Design review of the part built by this model. Coordinates are the model's own, in mm. Face numbers are marked on the shaded views. Coordinates: 2 decimals unless noted, no trailing zeros. Write each loop counter-clockwise with the first axis right and the second up, starting at its lowest first coordinate (ties: lowest second). Pieces come first, ordered by that corner, then holes. Notation, with made-up numbers: (-29, 54.5) -> (1, 54.5) arc R20 cw to (1, 90.5) -> close; hole circle Ø5 at (65, 21.25). An arc over 180 degrees is marked (long way). One line per question, with ' | ' between items. Start each with the question number.
Q1. For P1, Ø1.7, axis at x = 51, z = -55.5, coming from the +Y side; P2, Ø3, axis at x = 9.56, z = -17.28, coming from the +Y side; P3, Ø5.5, axis at x = 51.46, z = -30.78, coming from the -Y side; P4, Ø1.2, axis at x = 22.5, y = 2.5, coming from the -Z side, all flat-tipped, find the tip position at first contact; note any pin that passes through.
Q2. Add section A-A on z = -41.5. State the section outline as (x, y) points.
Q3. Draft analysis for pull direction Y (two halves, no side actions). For the marked faces 1 and 2, state which applies: pulls with the +Y half, pulls with the -Y half, needs draft (parallel to the pull), parting line crosses it, or undercut.
Q4. Wall thickness on probe 1 along X at (y, z) = (1.8, -15); probe 2 along X at (y, z) = (0.4, -55.5); probe 3 along X at (y, z) = (1.5, -41.5): over which ranges is each line inside the solid? List them lowest first.
Q5. Add section B-B on y = 2.65. State the section outline as (x, z) points.
Q6. Add section D-D on z = -18. State the section outline as (x, y) points, and give its area (3 significant figures).
Q7. Add section C-C on x = 21. State the section outline as (y, z) points.
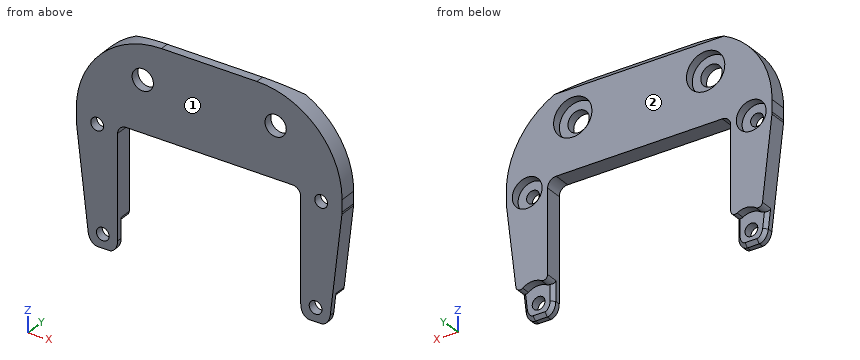
from build123d import *

# Parameters (mm, degrees)
SZKIC1_R                    = 1.5
SZKIC1_R_2                  = 2.5
DODANIE_WYCI_GNI_CIE1_DEPTH = 4
ZAOKR_GLENIE1_R             = 20
SZKIC2_R                    = 3.5
SZKIC2_R_2                  = 4
SZKIC2_R_3                  = 4.5
WYTNIJ_WYCI_GNI_CIE1_DEPTH  = 2
ZAOKR_GLENIE2_R             = 1
SFAZOWANIE2_SIZE            = 0.8


with BuildPart() as part:
    # Szkic1 → Dodanie-wyciągnięcie1 (new body)
    with BuildSketch(Plane(origin=(0, 0, 0), x_dir=(1, 0, 0), z_dir=(0, 1, 0))):
        with BuildLine():
            Line((1.659006671, 58.277593275), (-1.119868317, 58.277593275))
            add(Edge.make_bspline(
                [(-1.119868317, 58.277593275), (-2.968900305, 58.277593275), (-3.270926516, 55.680167866)],
                knots=[3.223355162, 3.223355162, 3.223355162, 4.71238898, 4.71238898, 4.71238898], degree=2, weights=[1, 0.735415338, 1]))
            Line((-3.270926516, 55.680167866), (-6.019830139, 32.039596707))
            ThreePointArc((-6.019830139, 32.039596707), (-6.039902389, 31.808982465), (-6.046600617, 31.577593275))
            Line((-6.046600617, 31.577593275), (-6.046600617, 8.777593275))
            Line((-6.046600617, 8.777593275), (56.36461396, 8.777593275))
            Line((56.36461396, 8.777593275), (56.36461396, 31.577593275))
            ThreePointArc((56.36461396, 31.577593275), (56.357915732, 31.808982465), (56.337843482, 32.039596707))
            Line((56.337843482, 32.039596707), (53.588939858, 55.680167866))
            add(Edge.make_bspline(
                [(53.588939858, 55.680167866), (53.286913648, 58.277593275), (51.43788166, 58.277593275)],
                knots=[1.570796327, 1.570796327, 1.570796327, 3.059830145, 3.059830145, 3.059830145], degree=2, weights=[1, 0.735415338, 1]))
            Line((51.43788166, 58.277593275), (48.659006671, 58.277593275))
            add(Edge.make_bspline(
                [(48.659006671, 58.277593275), (46.659006671, 58.277593275), (46.659006671, 55.44916615)],
                knots=[3.141592654, 3.141592654, 3.141592654, 4.71238898, 4.71238898, 4.71238898], degree=2, weights=[1, 0.707106781, 1]))
            Line((46.659006671, 55.44916615), (46.659006671, 31.277593275))
            ThreePointArc((46.659006671, 31.277593275), (46.073220234, 29.863379712), (44.659006671, 29.277593275))
            Line((44.659006671, 29.277593275), (5.659006671, 29.277593275))
            ThreePointArc((5.659006671, 29.277593275), (4.244793109, 29.863379712), (3.659006671, 31.277593275))
            Line((3.659006671, 31.277593275), (3.659006671, 55.44916615))
            add(Edge.make_bspline(
                [(3.659006671, 55.44916615), (3.659006671, 58.277593275), (1.659006671, 58.277593275)],
                knots=[1.570796327, 1.570796327, 1.570796327, 3.141592654, 3.141592654, 3.141592654], degree=2, weights=[1, 0.707106781, 1]))
        make_face()
        with Locations(Location((50.145621432, 55.076817676, 0), (0, 0, 270))):
            Circle(SZKIC1_R, mode=Mode.SUBTRACT)
        with Locations(Location((0.172391911, 55.076817676, 0), (0, 0, 270))):
            Circle(SZKIC1_R, mode=Mode.SUBTRACT)
        with Locations(Location((-1.144922446, 30.775394297, 0), (0, 0, 270))):
            Circle(SZKIC1_R, mode=Mode.SUBTRACT)
        with Locations(Location((51.462935789, 30.775394297, 0), (0, 0, 270))):
            Circle(SZKIC1_R, mode=Mode.SUBTRACT)
        with Locations(Location((40.761810316, 17.277593275, 0), (0, 0, 270))):
            Circle(SZKIC1_R_2, mode=Mode.SUBTRACT)
        with Locations(Location((9.556203027, 17.277593275, 0), (0, 0, 90))):
            Circle(SZKIC1_R_2, mode=Mode.SUBTRACT)
    extrude(amount=DODANIE_WYCI_GNI_CIE1_DEPTH)

    # Zaokrąglenie1
    zaokr_glenie1_edges = [part.edges().sort_by_distance(p)[0] for p in [
        (56.36461396, 2, -8.777593275),
        (-6.046600617, 2, -8.777593275),
    ]]
    fillet(zaokr_glenie1_edges, radius=ZAOKR_GLENIE1_R)

    # Szkic2 → Wytnij-wyciągnięcie1 (cut)
    with BuildSketch(Plane(origin=(0, 4, 0), x_dir=(1, 0, 0), z_dir=(0, 1, 0))):
        with Locations(Location((51.462935789, 30.775394297, 0), (0, 0, 270))):
            Circle(SZKIC2_R)
        with Locations((50.145621432, 55.076817676)):
            Circle(SZKIC2_R_2)
        with Locations((0.172391911, 55.076817676)):
            Circle(SZKIC2_R_2)
        with Locations(Location((-1.144922446, 30.775394297, 0), (0, 0, 270))):
            Circle(SZKIC2_R)
        with Locations(Location((9.556203027, 17.277593275, 0), (0, 0, 270))):
            Circle(SZKIC2_R_3)
        with Locations(Location((40.761810316, 17.277593275, 0), (0, 0, 270))):
            Circle(SZKIC2_R_3)
    extrude(amount=-WYTNIJ_WYCI_GNI_CIE1_DEPTH, mode=Mode.SUBTRACT)

    # Zaokrąglenie2
    zaokr_glenie2_edges = [part.edges().sort_by_distance(p)[0] for p in [
        (53.837974946, 3, -53.538466114),
        (-3.519961603, 3, -53.538466114),
        (3.659006671, 3, -53.116328576),
        (46.659006671, 3, -53.116328576),
    ]]
    fillet(zaokr_glenie2_edges, radius=ZAOKR_GLENIE2_R)

    # Sfazowanie1
    # the kernel refuses this chamfer: 2 mm, written as the material it takes off along each edge
    with BuildSketch(Plane(origin=(1.60932104, 4, -8.777593275), x_dir=(0, 0.027495876610586487, -0.9996219169112968), z_dir=(1, 0, 0))) as sfazowanie1_piece_1:
        with BuildLine():
            Line((2.05734639, 0), (-0.11309431, -2.054235587))
            Line((-0.11309431, -2.054235587), (-0.153079186, -2.053135752))
            ThreePointArc((-0.153079186, -2.053135752), (-0.068258454, -1.026795659), (-0.039984877, 0.001099835))
            Line((-0.039984877, 0.001099835), (0.001099835, 0.039984877))
            ThreePointArc((0.001099835, 0.039984877), (1.028995329, 0.011711299), (2.058446225, 0.039984877))
            Line((2.058446225, 0.039984877), (2.05734639, 0))
        make_face()
    extrude(amount=47.099371262, mode=Mode.SUBTRACT)

    # Sfazowanie2
    sfazowanie2_edges = [part.edges().sort_by_distance(p)[0] for p in [
        (3.659006671, 2, -53.094078185),
        (-3.532969865, 2, -53.426595059),
        (3.185598698, 2, -57.276468397),
        (-2.638843717, 2, -57.379483489),
        (0.269569177, 2, -58.277593275),
        (53.850983208, 2, -53.426595059),
        (46.659006671, 2, -53.094078185),
        (52.95685706, 2, -57.37948349),
        (47.132414645, 2, -57.276468396),
        (50.048444166, 2, -58.277593275),
    ]]
    chamfer(sfazowanie2_edges, length=SFAZOWANIE2_SIZE)


solid = part.part
Output values:
1) P1: stops at y = 2 | P2: passes through | P3: stops at y = 0 | P4: stops at z = -29.28
2) outline: (-4.92, 0) -> (3.66, 0) -> (3.66, 4) -> (-4.92, 4) -> close; (46.66, 0) -> (55.24, 0) -> (55.24, 4) -> (46.66, 4) -> close
3) face 1: pulls with the -Y half | face 2: pulls with the +Y half
4) probe 1: x = -0.54 to 8.53, 10.59 to 39.73, 41.79 to 50.86 | probe 2: x = -3.29 to -1.27, 1.61 to 3.66, 46.66 to 48.71, 51.58 to 53.61 | probe 3: x = -4.92 to 3.66, 46.66 to 55.24
5) outline: (-6.05, -31.58) arc R4 ccw to (-6.02, -32.04) -> (-3.8, -51.17) arc R1 ccw to (-2.21, -51.86) arc R4 cw to (2.16, -51.61) arc R1 ccw to (3.66, -50.74) -> (3.66, -31.28) arc R2 cw to (5.66, -29.28) -> (44.66, -29.28) arc R2 cw to (46.66, -31.28) -> (46.66, -50.74) arc R1 ccw to (48.16, -51.61) arc R4 cw to (52.52, -51.86) arc R1 ccw to (54.11, -51.17) -> (56.34, -32.04) arc R4 ccw to (56.36, -31.58) -> (56.36, -28.78) arc R20 ccw to (41.42, -9.43) -> (8.9, -9.43) arc R20 ccw to (-6.05, -28.78) -> close; hole circle Ø7 at (-1.14, -30.78); hole circle Ø9 at (9.56, -17.28); hole circle Ø9 at (40.76, -17.28); hole circle Ø7 at (51.46, -30.78)
6) outline: (-2.89, 0) -> (7.16, 0) -> (7.16, 2) -> (5.11, 2) -> (5.11, 4) -> (-2.89, 4) -> close; (11.95, 0) -> (38.37, 0) -> (38.37, 2) -> (36.32, 2) -> (36.32, 4) -> (14, 4) -> (14, 2) -> (11.95, 2) -> close; (43.16, 0) -> (53.21, 0) -> (53.21, 4) -> (45.2, 4) -> (45.2, 2) -> (43.16, 2) -> close | area: 170 mm2
7) outline: (0, -29.28) -> (4, -29.28) -> (4, -10.78) -> (2, -8.78) -> (0, -8.78) -> close
